Geometry check sheet. Reference: the model listing, model coordinates, mm. Face numbers are marked on the shaded views. A direction names the side the tool comes from. Give positions to 0.01 mm unless a question says otherwise; leave off trailing zeros. Write each question's results on one line, items separated by ' | '. Start each with the question number.
1) Scan lines: line 1 (X direction, y = 0, z = 27.75) (3 decimals); line 2 (Y direction, x = -76, z = 26); line 3 (Z direction, x = -31.5, y = 6.5). Record each from-to range of solid material in increasing order. Write a range as from..to.
2) Depth check by flat-ended pin: pin 1 (2 mm diameter, centred on y = 43, z = 15.5, fed in from +X); pin 2 (4 mm diameter, centred on x = -76.2, y = 0, fed in from -Z); pin 3 (2 mm diameter, centred on y = 55.5, z = -11.5, fed in from +X); pin 4 (6 mm diameter, centred on x = -41, z = 29, fed in from -Y). Enter the tip coordinate at first touch or a pass-through.
3) Set-up check for the marked faces 5 and 6: record each of +Z, -Z, +X, -X, +Y, -Y from which the full face is reachable in a straight line by a thin tool's end or side.
4) Draft check along Z on the marked faces 1, 2, 3 and 4. Enter one of: pulls with the +Z half, pulls with the -Z half, needs draft (parallel to the pull), parting line crosses it, or undercut.
```python
from build123d import *

# Parameters (mm, degrees)
SKETCH1_R           = 3.175
BOSS_EXTRUDE1_DEPTH = 39.37
SKETCH3_W           = 153.048335432
SKETCH3_H           = 25.4
CUT_EXTRUDE1_DEPTH  = 38.1
FILLET1_R           = 2.54
FILLET2_R           = 2.54


with BuildPart() as part:
    # Sketch1 → Boss-Extrude1 (new, symmetric)
    with BuildSketch(Plane.XY):
        with BuildLine():
            Line((-76.596875, -9.516728179), (-0.529166667, -12.688970905))
            ThreePointArc((-0.529166667, -12.688970905), (9.239000565, -8.713832025), (12.636340451, 1.27))
            Line((12.636340451, 1.27), (6.318170226, 64.135))
            ThreePointArc((6.318170226, 64.135), (-0.08833437, 69.849385564), (-6.333390084, 63.95898807))
            ThreePointArc((-6.333390084, 63.95898807), (-28.602299903, 21.707467551), (-74.754015102, 9.414603161))
            ThreePointArc((-74.754015102, 9.414603161), (-85.680189052, 0.922843719), (-76.596875, -9.516728179))
        make_face()
        with Locations((-76.2, 0)):
            Circle(SKETCH1_R, mode=Mode.SUBTRACT)
        Circle(SKETCH1_R, mode=Mode.SUBTRACT)
    extrude(amount=BOSS_EXTRUDE1_DEPTH, both=True)

    # Sketch3 → Cut-Extrude1 (cut)
    with BuildSketch(Plane(origin=(-0.529166667, -12.688970905, 0), x_dir=(0.9991315673568165, -0.04166666666666664, 0), z_dir=(-0.04166666666666664, -0.9991315673568165, 0))):
        with Locations((-41.471397415, 0)):
            Rectangle(SKETCH3_W, SKETCH3_H)
    extrude(amount=-CUT_EXTRUDE1_DEPTH, mode=Mode.SUBTRACT)

    # Fillet1
    fillet1_edges = [part.edges().sort_by_distance(p)[0] for p in [
        (-23.382807479, 26.397207842, 0),
        (10.25193425, 24.994542149, 0),
    ]]
    fillet(fillet1_edges, radius=FILLET1_R)

    # Fillet2
    fillet2_edges = [part.edges().sort_by_distance(p)[0] for p in [
        (-0.08833437, 69.849385564, 39.37),
        (-28.602299903, 21.707467551, 39.37),
        (-85.680189052, 0.922843719, 39.37),
        (-38.563020833, -11.102849542, 39.37),
        (9.239000565, -8.713832025, 39.37),
        (-38.563020833, -11.102849542, -39.37),
        (-85.680189052, 0.922843719, -39.37),
        (-28.602299903, 21.707467551, -39.37),
        (9.477255338, 32.7025, 39.37),
        (-0.08833437, 69.849385564, -39.37),
        (9.477255338, 32.7025, -39.37),
        (9.239000565, -8.713832025, -39.37),
    ]]
    fillet(fillet2_edges, radius=FILLET2_R)


solid = part.part
```
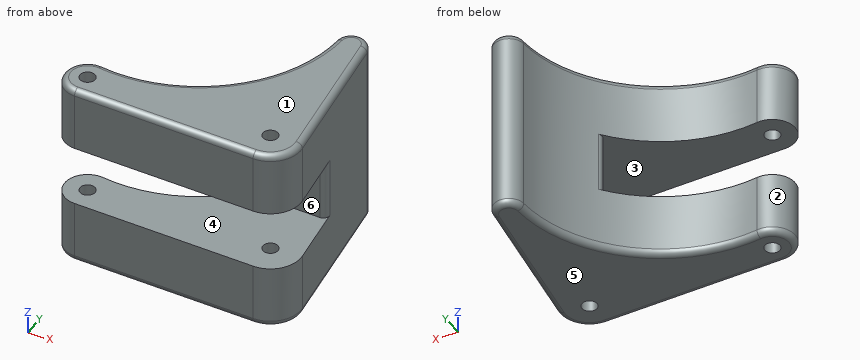
Result:
1) line 1: -85.725..-79.375, -73.025..-3.175, 3.175..12.7 | line 2: -9.54..-3.17, 3.17..9.52 | line 3: -39.37..-12.7, 12.7..39.37
2) pin 1: x = 8.54 | pin 2: through | pin 3: x = 7.29 | pin 4: y = -11.13
3) face 5: -Z, +X, -X, +Y, -Y | face 6: -X, -Y
4) face 1: pulls with the +Z half | face 2: needs draft | face 3: undercut | face 4: undercut
